```python
from build123d import *

# Parameters (mm, degrees)
ESQUISSE1_R             = 9
BOSS_EXTRU_1_DEPTH      = 19.075
ESQUISSE2_R             = 11.025
ENL_V_MAT_EXTRU_1_DEPTH = 5.5
ESQUISSE6_R             = 2
ENL_V_MAT_EXTRU_5_DEPTH = 6


with BuildPart() as part:
    # Esquisse1 → Boss.-Extru.1 (new body)
    with BuildSketch(Plane.XY):
        with BuildLine():
            Line((-56.5, 0), (-56.5, 5))
            Line((-56.5, 5), (-44.5, 5))
            Line((-44.5, 5), (-13.11591162, 49.70725189))
            ThreePointArc((-13.11591162, 49.70725189), (0, 56.525), (13.11591162, 49.70725189))
            Line((13.11591162, 49.70725189), (44.5, 5))
            Line((44.5, 5), (56.5, 5))
            Line((56.5, 5), (56.5, 0))
            Line((56.5, 0), (35.791970863, 0))
            Line((35.791970863, 0), (21.7521509, 20))
            Line((21.7521509, 20), (-21.7521509, 20))
            Line((-21.7521509, 20), (-35.791970863, 0))
            Line((-35.791970863, 0), (-56.5, 0))
        make_face()
        with Locations((0, 40.5)):
            Circle(ESQUISSE1_R, mode=Mode.SUBTRACT)
        with BuildLine():
            Line((-17.087305896, 35.347543053), (-25.844479018, 22.872777501))
            Line((-25.844479018, 22.872777501), (-3.323305878, 22.872777501))
            Line((-3.323305878, 22.872777501), (-3.323305878, 25.872777501))
            ThreePointArc((-3.323305878, 25.872777501), (-9.910860011, 29.240566007), (-14.087305896, 35.347543053))
            Line((-14.087305896, 35.347543053), (-17.087305896, 35.347543053))
        make_face(mode=Mode.SUBTRACT)
        with BuildLine():
            Line((17.087305896, 35.347543053), (25.844479018, 22.872777501))
            Line((25.844479018, 22.872777501), (3.323305878, 22.872777501))
            Line((3.323305878, 22.872777501), (3.323305878, 25.872777501))
            ThreePointArc((3.323305878, 25.872777501), (9.910860011, 29.240566007), (14.087305896, 35.347543053))
            Line((14.087305896, 35.347543053), (17.087305896, 35.347543053))
        make_face(mode=Mode.SUBTRACT)
    extrude(amount=BOSS_EXTRU_1_DEPTH)

    # Esquisse2 → Enlèv. mat.-Extru.1 (cut)
    with BuildSketch(Plane(origin=(0, 0, 0), x_dir=(-1, 0, 0), z_dir=(0, 0, -1))):
        with Locations((0, 40.5)):
            Circle(ESQUISSE2_R)
    extrude(amount=-ENL_V_MAT_EXTRU_1_DEPTH, mode=Mode.SUBTRACT)

    # Esquisse6 → Enlèv. mat.-Extru.5 (cut, through all)
    with BuildSketch(Plane(origin=(0, 5, 0), x_dir=(1, 0, 0), z_dir=(0, 1, 0))):
        with Locations(Location((-51.5, -4.5375, 0), (0, 0, 180))):  # turned: the seam where the file's is
            Circle(ESQUISSE6_R)
        with Locations((51.5, -4.5375)):
            Circle(ESQUISSE6_R)
        with Locations(Location((51.5, -14.5375, 0), (0, 0, 180))):  # turned: the seam where the file's is
            Circle(ESQUISSE6_R)
        with Locations((-51.5, -14.5375)):
            Circle(ESQUISSE6_R)
    extrude(amount=-ENL_V_MAT_EXTRU_5_DEPTH, mode=Mode.SUBTRACT)


solid = part.part
```
Build history of the part. All positions in model axes, mm. A direction names the side the tool comes from. Give positions to 0.01 mm unless a question says otherwise; leave off trailing zeros. Loops run counter-clockwise (first coordinate to the right, second up) from the corner with the lowest first, then second, coordinate; pieces in that order, holes last.
1) Band-saw the part on D-D on y = 44.5. List the corners of the cut face in (x, z) (3 decimals).
Values follow:
outline: (-16.771, 0) - (-10.274, 0) - (-10.274, 5.5) - (-8.062, 5.5) - (-8.062, 19.075) - (-16.771, 19.075) - close; (8.062, 5.5) - (10.274, 5.5) - (10.274, 0) - (16.771, 0) - (16.771, 19.075) - (8.062, 19.075) - close
2) Band-saw the part on C-C on z = 11.5. List the corners of the cut face in (x, y) (3 decimals), then the cut area to 3 significant figures.
Values follow:
outline: (-56.5, 0) - (-35.792, 0) - (-21.752, 20) - (21.752, 20) - (35.792, 0) - (56.5, 0) - (56.5, 5) - (44.5, 5) - (13.116, 49.707) arc R16.025 ccw to (-13.116, 49.707) - (-44.5, 5) - (-56.5, 5) - close; hole (-25.844, 22.873) - (-3.323, 22.873) - (-3.323, 25.873) arc R15 cw to (-14.087, 35.348) - (-17.087, 35.348) - close; hole circle Ø18 at (0, 40.5); hole (3.323, 22.873) - (25.844, 22.873) - (17.087, 35.348) - (14.087, 35.348) arc R15 cw to (3.323, 25.873) - close
area: 1,550 mm2
3) Two-plate mould, pull along Y, no slides. Class faces 1 (the face through (-0.215, 56.524, 9.404)), 2 (the face through (-53.347, 2.535, 3.771)), 3 (the face through (-16, 35.348, 9)): released by +Y, released by -Y, zero draft, split by the parting line, or undercut.
Values follow:
face 1: released by +Y
face 2: zero draft
face 3: undercut
4) Drop flat-ended pins along their axis: P1, Ø2, axis at x = -0.5, z = 12, coming from the -Y side; P2, Ø0.9, axis at y = 24.5, z = 5.5, coming from the +X side; P3, Ø4, axis at y = 42, z = 8, coming from the -X side; P4, Ø2.5, axis at x = 51.5, z = 4.54, coming from the -Y side. Give the stop position or say it passes through.
Values follow:
P1: stops at y = 20
P2: stops at x = 31.13
P3: stops at x = -19.93
P4: passes through
5) 3-axis set-ups, long thin cutter, end or side, ignore diameter. For faces 4 (the face through (49.5, 2.54, 4.45)), 5 (the face through (46, 0, 9)), 6 (the face through (-21.405, 29.197, 9.404)), 7 (the face through (1.44, 51.43, 2.71)), 8 (the face through (-28.7, 10.1, 9.4)): which of +Z, -Z, +X, -X, +Y, -Y reach the whole face in a straight line?
Values follow:
face 4: +Y, -Y
face 5: +Z, -Z, +X, -X, -Y
face 6: +Z, -Z
face 7: -Z
face 8: +Z, -Z, -Y
6) Probe line 1 along Z through (x, y) = (-51.5, 2.75) (1 decimal); line 2 along Z through (x, y) = (-51, 2) (3 decimals); line 3 along Y through (x, z) = (-4.5, 14.75). List the from-to ranges inside material, lowest first.
Values follow:
line 1: z = 0 to 2.5, 6.5 to 12.5, 16.5 to 19.1
line 2: z = 0 to 2.601, 6.474 to 12.601, 16.474 to 19.075
line 3: y = 20 to 22.87, 26.19 to 32.71, 48.29 to 55.88
7) Band-saw the part on B-B on x = 51.5. List the corners of the cut face in (y, z) (1 decimal).
Values follow:
outline: (0, 0) - (5, 0) - (5, 2.5) - (0, 2.5) - close; (0, 6.5) - (5, 6.5) - (5, 12.5) - (0, 12.5) - close; (0, 16.5) - (5, 16.5) - (5, 19.1) - (0, 19.1) - close
8) Band-saw the part on A-A on x = 0. List the corners of the cut face in (y, z) (3 decimals), then the cut area to 3 significant figures.
Values follow:
outline: (20, 0) - (29.475, 0) - (29.475, 5.5) - (31.5, 5.5) - (31.5, 19.075) - (20, 19.075) - close; (49.5, 5.5) - (51.525, 5.5) - (51.525, 0) - (56.525, 0) - (56.525, 19.075) - (49.5, 19.075) - close
area: 331 mm2
